CAD build for the part. Positions are in the model's coordinates, mm. Face numbers are marked on the shaded views. A direction names the side the tool comes from. Round coordinates to 2 decimals unless told otherwise and drop trailing zeros. Loops run counter-clockwise (first coordinate to the right, second up) from the corner with the lowest first, then second, coordinate; pieces in that order, holes last. Notation, with made-up numbers: M -23.5,-36 L -4.5,-36 A19 ccw -4.5,-30 Z; hole C -38.5,-9.75 d10. An arc over 180 degrees is marked long. Use one line per item in the form item = value.
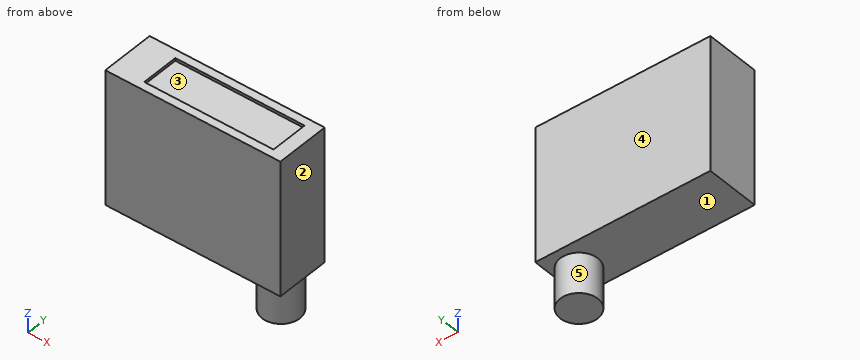
from build123d import *

# Parameters (mm, degrees)
SKETCH2_W           = 65
SKETCH2_H           = 50
BOSS_EXTRUDE1_DEPTH = 20
SKETCH3_R           = 7
BOSS_EXTRUDE2_DEPTH = 15
SKETCH4_W           = 48
SKETCH4_H           = 14
CUT_EXTRUDE1_DEPTH  = 1


with BuildPart() as part:
    # Sketch2 → Boss-Extrude1 (new body)
    with BuildSketch(Plane(origin=(0, 0, 0), x_dir=(1, 0, 0), z_dir=(0, 1, 0))):
        Rectangle(SKETCH2_W, SKETCH2_H)
    extrude(amount=BOSS_EXTRUDE1_DEPTH)

    # Sketch3 → Boss-Extrude2 (add)
    with BuildSketch(Plane(origin=(0, 0, -25), x_dir=(-1, 0, 0), z_dir=(0, 0, -1))):
        with Locations(Location((-24.5, 10, 0), (0, 0, 180))):
            Circle(SKETCH3_R)
    extrude(amount=BOSS_EXTRUDE2_DEPTH)

    # Sketch4 → Cut-Extrude1 (cut)
    with BuildSketch(Plane.XY.offset(25)):
        with Locations((3.5, 10)):
            Rectangle(SKETCH4_W, SKETCH4_H)
    extrude(amount=-CUT_EXTRUDE1_DEPTH, mode=Mode.SUBTRACT)


solid = part.part
1. Pull direction X, two halves, no side cores. Call the marked faces 1, 2 and 3: +X half, -X half, draft (parallel to the pull), parting line (faces both ways), or undercut.
Completed:
face_1 = draft
face_2 = +X half
face_3 = undercut
2. Cut at C-C on z = -31. Write the cut outline in (x, y), and give its area (3 significant figures).
Completed:
outline = C 24.5,10 d14
area = 154 mm2
3. Drop flat-ended pins along their axis: P1, Ø6, axis at x = -3.5, y = 13, coming from the -Z side; P2, Ø4, axis at x = -2.5, y = 6.5, coming from the +Z side. Give the stop position or say it passes through.
Completed:
P1 = -25
P2 = 24
4. Cut at D-D on x = 24.5. Write the cut outline in (y, z), and give its area (3 significant figures).
Completed:
outline = M 0,-25 L 3,-25 L 3,-40 L 17,-40 L 17,-25 L 20,-25 L 20,25 L 17,25 L 17,24 L 3,24 L 3,25 L 0,25 Z
area = 1,200 mm2
5. Cut at B-B on y = 10. Write the cut outline in (x, z), and give its area (3 significant figures).
Completed:
outline = M -32.5,-25 L 17.5,-25 L 17.5,-40 L 31.5,-40 L 31.5,-25 L 32.5,-25 L 32.5,25 L 27.5,25 L 27.5,24 L -20.5,24 L -20.5,25 L -32.5,25 Z
area = 3,410 mm2
6. Probe line 1 along Z through (x, y) = (4.5, 14.75); line 2 along Z through (x, y) = (7, 17.25); line 3 along X through (y, z) = (9.75, -33). List the from-to ranges inside material, lowest first. Write a range as from..to.
Completed:
line_1 = -25..24
line_2 = -25..25
line_3 = 17.5..31.5
7. Tool access for the marked faces 4 and 5: list every direction of +Z, -Z, +X, -X, +Y, -Y with a clear straight run to the whole face (end or side of a thin tool).
Completed:
face_4 = +Z, -Z, +X, -X, +Y
face_5 = -Z
8. Cut at A-A on x = -12.5. Write the cut outline in (y, z).
Completed:
outline = M 0,-25 L 20,-25 L 20,25 L 17,25 L 17,24 L 3,24 L 3,25 L 0,25 Z
